from build123d import *

# Parameters (mm, degrees)
HEX_2_DEPTH                 = 2.5
TAP_DRILL_FOR_M3X0_5_TAP1_D = 2.5
INNERCHAMFER_SIZE           = 0.25


with BuildPart() as part:
    # Sketch1 → HEX 2 (new body, symmetric)
    with BuildSketch(Plane.XY):
        Polygon((2.886751346, 0), (1.443375673, 2.5), (-1.443375673, 2.5), (-2.886751346, 0), (-1.443375673, -2.5), (1.443375673, -2.5), align=None)
    extrude(amount=HEX_2_DEPTH, both=True)

    # Tap Drill for M3x0.5 Tap1 (through all)
    with Locations(Plane.XY.offset(2.5)):
        with Locations((0, 0)):
            Hole(TAP_DRILL_FOR_M3X0_5_TAP1_D / 2)

    # Sketch7 → HexChamfer (revolve, cut)
    with BuildSketch(Plane(origin=(0, 0, 0), x_dir=(1, 0, 0), z_dir=(0, 1, 0))):
        Polygon((-2.886751346, 2.5), (-2.886751346, 2.1), (-2.486751346, 2.5), align=None)
    hexchamfer = revolve(axis=Axis((0, 0, 15.266742202), (0, 0, -1)), mode=Mode.SUBTRACT)

    # Mirror1: HexChamfer across plane
    add(hexchamfer.mirror(Plane.XY), mode=Mode.SUBTRACT)

    # InnerChamfer
    innerchamfer_edges = [part.edges().sort_by_distance(p)[0] for p in [
        (1.25, 0, 2.5),
        (1.25, 0, -2.5),
    ]]
    chamfer(innerchamfer_edges, length=INNERCHAMFER_SIZE)


solid = part.part
Design review of the part built by this model. Coordinates are the model's own, in mm. Give positions to 0.01 mm unless a question says otherwise; leave off trailing zeros. Order: outer loops, then holes, each group sorted by start corner. A loop starts at its lowest first (then second) coordinate and runs counter-clockwise, first axis right, second up.
1. To check wall thickness, follow L1, parallel to Y at x = 0, z = 0.7; L2, parallel to Y at x = 1.1, z = -0.25; L3, parallel to Z at x = -1.3, y = 2.25. State the ranges of each line that lie inside material, in increasing order.
Solution:
L1: y = -2.5 to -1.25, 1.25 to 2.5
L2: y = -2.5 to -0.59, 0.59 to 2.5
L3: z = -2.39 to 2.39
2. Add section A-A, the plane z = -0.1. State the section outline as (x, y) points.
Solution:
outline: (-2.89, 0) - (-1.44, -2.5) - (1.44, -2.5) - (2.89, 0) - (1.44, 2.5) - (-1.44, 2.5) - close; hole circle Ø2.5 at (0, 0)
3. For pin 1 Ø1.5 at (y, z) = (-0.5, 1.5) entering from -X, flat-tipped, find the tip position at first contact; note if it passes through.
Solution:
pin 1: stops at x = -2.89
4. Mouldability with a two-part tool opening along Y and no side actions: class faces 1 (the flat face through (2.175, 1.233, 0.035)), 2 (the flat face through (2.155, -1.268, 0.035)), 3 (the cylindrical face through (0.27, -1.22, -0.03)) as +Y half, -Y half, draft (parallel to the pull), parting line (faces both ways), or undercut.
Solution:
face 1: +Y half
face 2: -Y half
face 3: undercut
